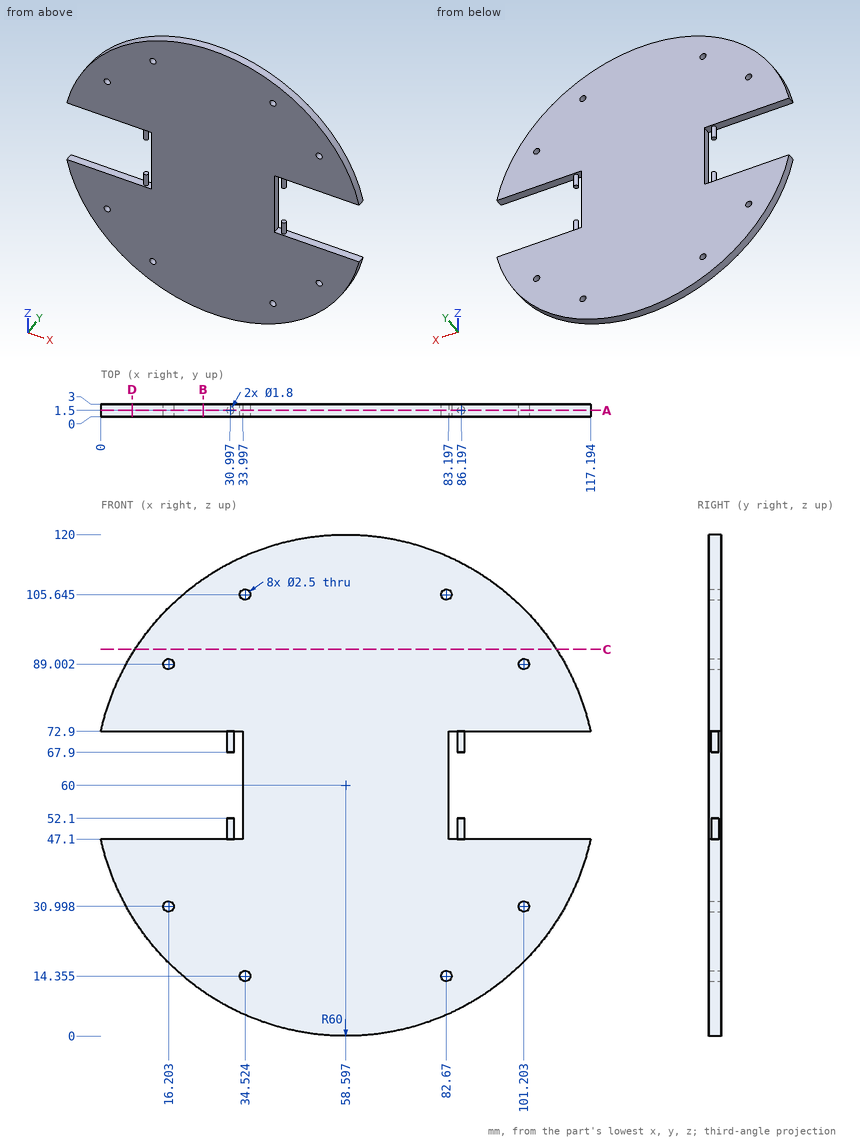
Here's the drawing with two shaded views (mm, measured from the low corner). I have some questions. Give positions to 0.01 mm unless a question says otherwise; leave off trailing zeros. Write each loop counter-clockwise with the first axis right and the second up, starting at its lowest first coordinate (ties: lowest second). Pieces come first, ordered by that corner, then holes. Notation, with made-up numbers: (-21, 25) - (-3, 25) arc R22 ccw to (-3, 32) - close; hole circle Ø2 at (20.5, 65.5). An arc over 180 degrees is marked (long way). One line per item, written item: value. Start each with the question number.
Item 1: Imagine slicing it at C-C, the plane z = 92.5. List the corners of the cut face in (x, y) for me.
Item 2: Imagine slicing it at D-D, the plane x = 7.5. List the corners of the cut face in (y, z) for me.
Item 3: I'm going to push flat-ended pins straight in: pin 1 (0.5 mm diameter, centred on x = 31.5, y = 1, fed in from -Z); pin 2 (1.4 mm diameter, centred on x = 31, y = 2, fed in from +Z); pin 3 (1 mm diameter, centred on y = 2, z = 102, fed in from -X) (1 decimal). Where does each tip first touch, or does it pass through?
Item 4: Imagine slicing it at A-A, the plane y = 1.5. Give the number of separate pieces and of enclosed holes in the cut face, and give its area (3 significant figures).
Item 5: Please list where these lines run through material, in increasing order: line 1 (X direction, y = 1.6, z = 48.5); line 2 (X direction, y = 1.35, z = 73); line 3 (Z direction, x = 109, y = 0.1). Write a range as from..to.
Item 6: Imagine slicing it at B-B, the plane x = 24.5. List the corners of the cut face in (y, z) for me, and give its area (3 significant figures).
Geometry says:
1. outline: (8.16, 0) - (109.03, 0) - (109.03, 3) - (8.16, 3) - close
2. outline: (0, 28.55) - (3, 28.55) - (3, 47.1) - (0, 47.1) - close; (0, 72.9) - (3, 72.9) - (3, 91.45) - (0, 91.45) - close
3. pin 1: z = 6.34
3. pin 2: z = 113.63
3. pin 3: x = 15.3
4. separate pieces: 1
4. enclosed holes: 8
4. area: 9,500 mm^2
5. line 1: 30.1..31.89, 34..83.2, 85.3..87.09
5. line 2: 0.02..117.17
5. line 3: 27.45..47.1, 72.9..92.55
6. outline: (0, 10.63) - (3, 10.63) - (3, 47.1) - (0, 47.1) - close; (0, 72.9) - (3, 72.9) - (3, 109.37) - (0, 109.37) - close
6. area: 219 mm^2
